Check sheet for the modelled part. Datum: model origin and axes. Units: mm. A direction names the side the tool comes from. Round coordinates to 2 decimals unless told otherwise and drop trailing zeros. Loops run counter-clockwise (first coordinate to the right, second up) from the corner with the lowest first, then second, coordinate; pieces in that order, holes last. Notation, with made-up numbers: M -28,-30.5 L 29,-30.5 A18 ccw 29,-5.5 Z; hole C -17.5,-37 d6. An arc over 180 degrees is marked long. One line per question, with ' | ' between items. Start each with the question number.
(1) Thickness scan on probe 1 along Y at (x, z) = (0, 0.65); probe 2 along Z at (x, y) = (16.2, 0); probe 3 along Y at (x, z) = (-24, 1). Record the ranges inside material, lowest first. Write a range as [from, to].
(2) Section check A-A (z = -30). Record the boundary of the cut face in (x, y), and give its area (3 significant figures).
(3) Section check C-C (y = 0). Record the boundary of the cut face in (x, z), and give its area (3 significant figures).
(4) Section check D-D (z = -1.5). Record the boundary of the cut face in (x, y).
(5) Tool access check on faces 4 (the face through (11, -11, -12)), 5 (the face through (15.2, 0, -2)), 6 (the face through (16.186, 10.797, -16.641)). Record the directions out of +Z, -Z, +X, -X, +Y, -Y that give a thin tool (end or side, any length) a straight path to the whole face; none if there is none.
(6) Section check B-B (x = 0). Record the boundary of the cut face in (y, z).
(7) Draft check along Y on faces 1 (the face through (16.186, -10.797, -38.359)), 2 (the face through (-26, -14, -20)), 3 (the face through (-27, -12, -20)). Enter one of: +Y half, -Y half, draft (parallel to the pull), parting line (faces both ways), or undercut.
(8) Go/stop test with flat-tipped pins: P1, Ø1.5, axis at x = 4.5, y = 23, coming from the -Z side; P2, Ø2.5, axis at y = 0, z = -6.5, coming from the -X side; P3, Ø12, axis at x = 8, y = -4, coming from the -Z side; P4, Ø12, axis at y = 6, z = -36, coming from the -X side. Record where each tip stops, or that it passes through.
Autodesk Inventor part; units mm, degrees
ref_plane "YZ Plane" through (0, 0, 0) normal (1, 0, 0) x (0, 1, 0)
ref_plane "XZ Plane" through (0, 0, 0) normal (0, 1, 0) x (-1, 0, 0)
ref_plane "XY Plane" through (0, 0, 0) normal (0, 0, 1) x (1, 0, 0)
sketch "Sketch1" plane through (0, 0, 0) normal (0, 0, 1) x (1, 0, 0)
  circle A0 centre (0, 0) radius 15 construction
  line L0 (0, 0) -> (0, -12) construction
  line L1 (0, -12) -> (0, 28) construction
  line L2 (0, 28) -> (12, 28) construction
  line L3 (12, 28) -> (-28, 28) construction
  line L4 (-28, 28) -> (-28, -12) construction
  line L5 (-28, -12) -> (12, -12) construction
  line L6 (12, -12) -> (12, 28) construction
  line L7 (-28, 28) -> (17.2, 28)
  line L8 (17.2, 28) -> (17.2, -17.2)
  line L9 (17.2, -17.2) -> (-28, -17.2)
  line L10 (-28, -17.2) -> (-28, 28)
  circle A1 centre (0, 0) radius 15.25
  line L11 (0, -15.25) -> (0, -17.25) construction
  line L12 (-28, -17.2) -> (17.2, -17.2)
  line L13 (17.2, -17.2) -> (17.2, -15.3)
  line L14 (-28, -15.3) -> (-28, -17.2)
  line L15 (17.2, 28) -> (15.3, 28)
  line L16 (17.2, -15.3) -> (17.2, 28)
  circle A2 centre (0, 0) radius 16.85
  line L17 (15.25, 0) -> (17.25, 0) construction
  line L18 (-28, -17.2) -> (17.2, -17.2)
  line L19 (17.2, -17.2) -> (17.2, -15.2)
  line L20 (17.2, -15.2) -> (-28, -15.2)
  line L21 (-28, -15.2) -> (-28, -17.2)
  line L22 (17.2, -15.2) -> (15.2, -15.2)
  line L23 (15.2, -15.2) -> (15.2, 28)
  line L24 (15.2, 28) -> (17.2, 28)
  line L25 (17.2, 28) -> (17.2, -15.2)
  line L26 (-28, -12) -> (-26, -12)
  line L27 (-26, -12) -> (-26, -15.2)
  line L28 (-26, -15.2) -> (-28, -15.2)
  line L29 (-28, -15.2) -> (-28, -12)
  line L30 (15.2, 28) -> (12, 28)
  line L31 (12, 28) -> (12, 26)
  line L32 (12, 26) -> (15.2, 26)
  line L33 (15.2, 26) -> (15.2, 28)
  point P0 (15.2, -7.272)
  point P1 (15.2, 1.2339)
  point P2 (-1.2339, -15.2)
  point P3 (7.272, -15.2)
  point P4 (15.2, 7.272)
  point P5 (-7.272, -15.2)
  point P6 (15.2, -1.2339)
  point P7 (1.2339, -15.2)
  dimension "d0" = 30
  dimension "d1" = 12
  dimension "d2" = 40
  dimension "d3" = 12
  dimension "d4" = 40
  dimension "d5" = 40
  dimension "d6" = 45.2
  dimension "d7" = 45.2
  dimension "d8" = 30.5
  dimension "d22" = 2
  dimension "d30" = 1.6
  dimension "d33" = 2
  dimension "d34" = 2
  dimension "d35" = 2
  dimension "d43" = 2
  dimension "d44" = 2
extrude "Extrusion1" add sketch "Sketch1" along normal blind 2 contours L7 L31 L32 L23 A2 L20 L27 L26 L10 | L7 L23 L32 L31 | L26 L27 L20 L10 | L7 L8 L20 L23 A2 | L20 A2 L8 L9 L10 | L23 A1 L20 A2 | A2 L23 A1 | L20 A1 A2 | L20 A1 L23 A2 | A2 L23 L20
sketch "Sketch2" plane through (0, 0, 2) normal (0, 0, 1) x (1, 0, 0)
  line L0 (17.2, 28) -> (-28, 28) construction
  line L1 (-28, 28) -> (-28, 24) construction
  line L2 (-28, 28) -> (-28, -17.2) construction
  line L3 (-28, 24) -> (-24, 24) construction
  line L4 (-24, 24) -> (0, 24) construction
  line L5 (-24, 24) -> (-24, 0) construction
  point P0 (0, 0)
  dimension "d11" = 4
  dimension "d12" = 4
  dimension "d13" = 24
  dimension "d14" = 24
hole "Hole1" at (0, 24, 2) at (-24, 24, 2) at (-24, 0, 2) direction (0, 0, -1) diameter 4 end through all
extrude "Extrusion5" add sketch "Sketch1" against normal blind 41 contours L7 L8 L20 L23 A2 | L20 A2 L8 L9 L10 | A2 L23 A1 | L20 A1 A2 | A1 L23 | L20 A1
fillet "Fillet1" radius 1 3 edges at (-5.4, -17.2, 2) (17.2, 5.4, 2) (17.2, -17.2, -19.5)
extrude "Extrusion8" add sketch "Sketch1" against normal blind 41 contours L7 L23 L32 L31 | L26 L27 L20 L10
extrude "Extrusion12" add sketch "Sketch1" against normal blind 12 contours L23 A1 L20 A2 | L20 A1 L23 A2
sketch "Sketch5" plane through (17.2, -16.2, -41) normal (1, 0, 0) x (0, 0, -1)
  line L0 (0, 44.2) -> (0, 0) construction
  line L1 (0, 44.2) -> (0, 16.2) construction
  line L2 (0, 16.2) -> (-13.5, 16.2) construction
  line L3 (-41, 44.2) -> (-41, 42.2) construction
  line L4 (-41, 44.2) -> (-41, 16.2) construction
  line L5 (-41, 16.2) -> (-34.5, 16.2) construction
  circle A0 centre (-34.5, 16.2) radius 2
  line L6 (-25.5, 4.2) -> (-1.5, 4.2)
  line L7 (-1.5, 4.2) -> (-1.5, 28.2)
  line L8 (-1.5, 28.2) -> (-25.5, 28.2)
  line L9 (-25.5, 28.2) -> (-25.5, 4.2)
  line L10 (-25.5, 4.2) -> (-1.5, 28.2) construction
  line L11 (-1.5, 4.2) -> (-25.5, 28.2) construction
  dimension "d64" = 28
  dimension "d65" = 13.5
  dimension "d66" = 6.5
  dimension "d67" = 4
extrude "Extrusion14" cut sketch "Sketch5" against normal blind 3
fillet "Fillet2" radius 4 4 edges at (16.2, 12, -15.5) (16.2, -12, -15.5) (16.2, -12, -39.5) (16.2, 12, -39.5)
properties part number "MirrorFix" material "ABS Plastic"
The answers:
1) probe 1: [-17.2, -15.25], [15.25, 22], [26, 28] | probe 2: [-41, -39.5], [-15.5, -8.5], [-4.5, 2] | probe 3: [-17.2, -2], [2, 22], [26, 28]
2) outline: M -28,-17.2 L 16.2,-17.2 A1 ccw 17.2,-16.2 L 17.2,-12 L 15.2,-12 L 15.2,-15.2 L -26,-15.2 L -26,-12 L -28,-12 Z; M 12,26 L 15.2,26 L 15.2,12 L 17.2,12 L 17.2,28 L 12,28 Z | area: 141 mm²
3) outline: M -28,0 L -26,0 L -26,2 L -28,2 Z; M -22,0 L -16.85,0 L -16.85,-12 L -15.25,-12 L -15.25,2 L -22,2 Z; M 15.2,-41 L 17.2,-41 L 17.2,-39.5 L 15.2,-39.5 Z; M 15.2,-15.5 L 17.2,-15.5 L 17.2,-8.5 L 15.2,-8.5 Z; M 15.2,-4.5 L 17.2,-4.5 L 17.2,1 A1 ccw 16.2,2 L 15.25,2 L 15.25,0 L 15.2,0 Z | area: 66.4 mm²
4) outline: M -28,-17.2 L 16.2,-17.2 A1 ccw 17.2,-16.2 L 17.2,28 L 12,28 L 12,26 L 15.2,26 L 15.2,7.27 A16.85 ccw long -7.27,-15.2 L -26,-15.2 L -26,-12 L -28,-12 Z; hole M -1.23,-15.2 L 1.23,-15.2 A15.25 ccw 15.2,-1.23 L 15.2,1.23 A15.25 ccw long Z; hole M 7.27,-15.2 L 15.2,-15.2 L 15.2,-7.27 A16.85 cw Z
5) face 4: -Z | face 5: +Z, -Z | face 6: +X, -X
6) outline: M -17.2,-41 L -15.2,-41 L -15.2,0 L -15.25,0 L -15.25,2 L -16.2,2 A1 ccw -17.2,1 Z; M 15.25,-12 L 16.85,-12 L 16.85,0 L 22,0 L 22,2 L 15.25,2 Z; M 26,0 L 28,0 L 28,2 L 26,2 Z
7) face 1: undercut | face 2: draft | face 3: +Y half
8) P1: z = 0 | P2: x = -16.85 | P3: through | P4: x = 15.2
